```python
from build123d import *

# Parameters (mm, degrees)
SKETCH1_W                      = 42
SKETCH1_H                      = 42
BOSS_EXTRUDE1_DEPTH            = 22
CUT_EXTRUDE1_REACH             = 24
SKETCH2_R                      = 11.5
SKETCH2_R_2                    = 1.65
CUT_EXTRUDE1_DIRECTION_2_DEPTH = 1
CHAMFER1_SIZE                  = 4
SKETCH3_R                      = 3
CUT_EXTRUDE2_DEPTH             = 1
CUT_EXTRUDE2_DEPTH_BACK        = 5
CUT_EXTRUDE3_REACH             = 24
SKETCH4_R                      = 4.15
CUT_EXTRUDE3_DIRECTION_2_DEPTH = 1


with BuildPart() as part:
    # Sketch1 → Boss-Extrude1 (new body)
    with BuildSketch(Plane(origin=(0, 0, 0), x_dir=(1, 0, 0), z_dir=(0, 1, 0))):
        Rectangle(SKETCH1_W, SKETCH1_H)
    extrude(amount=BOSS_EXTRUDE1_DEPTH)

    # Sketch2 → Cut-Extrude1 (cut, up to next)
    with BuildSketch(Plane(origin=(0, 22, 0), x_dir=(1, 0, 0), z_dir=(0, 1, 0)), mode=Mode.PRIVATE) as cut_extrude1_sk1:
        Circle(SKETCH2_R)
    cut_extrude1_tool1 = extrude(cut_extrude1_sk1.sketch, amount=-CUT_EXTRUDE1_REACH, mode=Mode.PRIVATE) & part.part
    add(cut_extrude1_tool1.solids().sort_by_distance((0, 22, 0))[0], mode=Mode.SUBTRACT)
    # Sketch2 → Cut-Extrude1 (cut, up to next)
    with BuildSketch(Plane(origin=(0, 22, 0), x_dir=(1, 0, 0), z_dir=(0, 1, 0)), mode=Mode.PRIVATE) as cut_extrude1_sk2:
        with Locations((-15.5, 15)):
            Circle(SKETCH2_R_2)
    cut_extrude1_tool2 = extrude(cut_extrude1_sk2.sketch, amount=-CUT_EXTRUDE1_REACH, mode=Mode.PRIVATE) & part.part
    add(cut_extrude1_tool2.solids().sort_by_distance((-15.5, 22, -15))[0], mode=Mode.SUBTRACT)
    # Sketch2 → Cut-Extrude1 (cut, up to next)
    with BuildSketch(Plane(origin=(0, 22, 0), x_dir=(1, 0, 0), z_dir=(0, 1, 0)), mode=Mode.PRIVATE) as cut_extrude1_sk3:
        with Locations((15.5, 15)):
            Circle(SKETCH2_R_2)
    cut_extrude1_tool3 = extrude(cut_extrude1_sk3.sketch, amount=-CUT_EXTRUDE1_REACH, mode=Mode.PRIVATE) & part.part
    add(cut_extrude1_tool3.solids().sort_by_distance((15.5, 22, -15))[0], mode=Mode.SUBTRACT)
    # Sketch2 → Cut-Extrude1 (cut, up to next)
    with BuildSketch(Plane(origin=(0, 22, 0), x_dir=(1, 0, 0), z_dir=(0, 1, 0)), mode=Mode.PRIVATE) as cut_extrude1_sk4:
        with Locations((15.5, -15)):
            Circle(SKETCH2_R_2)
    cut_extrude1_tool4 = extrude(cut_extrude1_sk4.sketch, amount=-CUT_EXTRUDE1_REACH, mode=Mode.PRIVATE) & part.part
    add(cut_extrude1_tool4.solids().sort_by_distance((15.5, 22, 15))[0], mode=Mode.SUBTRACT)
    # Sketch2 → Cut-Extrude1 (cut, up to next)
    with BuildSketch(Plane(origin=(0, 22, 0), x_dir=(1, 0, 0), z_dir=(0, 1, 0)), mode=Mode.PRIVATE) as cut_extrude1_sk5:
        with Locations((-15.5, -15)):
            Circle(SKETCH2_R_2)
    cut_extrude1_tool5 = extrude(cut_extrude1_sk5.sketch, amount=-CUT_EXTRUDE1_REACH, mode=Mode.PRIVATE) & part.part
    add(cut_extrude1_tool5.solids().sort_by_distance((-15.5, 22, 15))[0], mode=Mode.SUBTRACT)

    # Sketch2 → Cut-Extrude1 direction 2 (cut)
    with BuildSketch(Plane(origin=(0, 22, 0), x_dir=(1, 0, 0), z_dir=(0, 1, 0))):
        Circle(SKETCH2_R)
        with Locations((-15.5, 15)):
            Circle(SKETCH2_R_2)
        with Locations((15.5, 15)):
            Circle(SKETCH2_R_2)
        with Locations((15.5, -15)):
            Circle(SKETCH2_R_2)
        with Locations((-15.5, -15)):
            Circle(SKETCH2_R_2)
    extrude(amount=CUT_EXTRUDE1_DIRECTION_2_DEPTH, mode=Mode.SUBTRACT)

    # Chamfer1
    chamfer1_edges = [part.edges().sort_by_distance(p)[0] for p in [
        (21, 11, 21),
        (-21, 11, 21),
        (-21, 11, -21),
        (21, 11, -21),
    ]]
    chamfer(chamfer1_edges, length=CHAMFER1_SIZE)

    # Sketch3 → Cut-Extrude2 (cut, two sides)
    with BuildSketch(Plane.XZ) as cut_extrude2_sk:
        with Locations((-15.5, 15)):
            Circle(SKETCH3_R)
        with Locations((15.5, 15)):
            Circle(SKETCH3_R)
        with Locations((15.5, -15)):
            Circle(SKETCH3_R)
        with Locations((-15.5, -15)):
            Circle(SKETCH3_R)
    extrude(amount=CUT_EXTRUDE2_DEPTH, mode=Mode.SUBTRACT)
    extrude(cut_extrude2_sk.sketch, amount=-CUT_EXTRUDE2_DEPTH_BACK, mode=Mode.SUBTRACT)

    # Sketch4 → Cut-Extrude3 (cut, up to next)
    with BuildSketch(Plane(origin=(0, 22, 0), x_dir=(1, 0, 0), z_dir=(0, 1, 0)), mode=Mode.PRIVATE) as cut_extrude3_sk1:
        with Locations((-21, 0)):
            Circle(SKETCH4_R)
    cut_extrude3_tool1 = extrude(cut_extrude3_sk1.sketch, amount=-CUT_EXTRUDE3_REACH, mode=Mode.PRIVATE) & part.part
    add(cut_extrude3_tool1.solids().sort_by_distance((-21, 22, 0))[0], mode=Mode.SUBTRACT)
    # Sketch4 → Cut-Extrude3 (cut, up to next)
    with BuildSketch(Plane(origin=(0, 22, 0), x_dir=(1, 0, 0), z_dir=(0, 1, 0)), mode=Mode.PRIVATE) as cut_extrude3_sk2:
        with Locations((21, 0)):
            Circle(SKETCH4_R)
    cut_extrude3_tool2 = extrude(cut_extrude3_sk2.sketch, amount=-CUT_EXTRUDE3_REACH, mode=Mode.PRIVATE) & part.part
    add(cut_extrude3_tool2.solids().sort_by_distance((21, 22, 0))[0], mode=Mode.SUBTRACT)

    # Sketch4 → Cut-Extrude3 direction 2 (cut)
    with BuildSketch(Plane(origin=(0, 22, 0), x_dir=(1, 0, 0), z_dir=(0, 1, 0))):
        with Locations((-21, 0)):
            Circle(SKETCH4_R)
        with Locations((21, 0)):
            Circle(SKETCH4_R)
    extrude(amount=CUT_EXTRUDE3_DIRECTION_2_DEPTH, mode=Mode.SUBTRACT)


solid = part.part
```
CAD build for the part. Positions are in the model's coordinates, mm. A direction names the side the tool comes from. Round coordinates to 2 decimals unless told otherwise and drop trailing zeros. Order: outer loops, then holes, each group sorted by start corner. A loop starts at its lowest first (then second) coordinate and runs counter-clockwise, first axis right, second up. Notation, with made-up numbers: (70, 56.5) -> (124, 56.5) arc R23 cw to (124, 81.5) -> close; hole circle Ø11 at (-5, 79). An arc over 180 degrees is marked (long way). One line per question, with ' | ' between items.
Q1. Two-plate mould, pull along Z, no slides. Class faces 3 (the cylindrical face through (17.074, 13.619, 14.504)), 4 (the flat face through (21, 11, -10)), 5 (the cylindrical face through (-13.926, 13.619, 14.504)), 6 (the flat face through (19, 11, -19)): released by +Z, released by -Z, zero draft, split by the parting line, or undercut.
Completed:
face 3: undercut | face 4: zero draft | face 5: undercut | face 6: released by -Z
Q2. Slice it at B-B (x = 0). Write the cut outline in (y, z), then the cut area to 3 significant figures.
Completed:
outline: (0, -21) -> (22, -21) -> (22, -11.5) -> (0, -11.5) -> close; (0, 11.5) -> (22, 11.5) -> (22, 21) -> (0, 21) -> close | area: 418 mm^2
Q3. Probe probe 1 along X at (y, z) = (14.25, 15); probe 2 along X at (y, z) = (5.5, -16.5); probe 3 along Z at (x, y) = (15, 12.25). List the from-to ranges inside material, lowest first.
Completed:
probe 1: x = -21 to -17.15, -13.85 to 13.85, 17.15 to 21 | probe 2: x = -21 to -16.19, -14.81 to 14.81, 16.19 to 21 | probe 3: z = -21 to -16.57, -13.43 to 13.43, 16.57 to 21
Q4. Slice it at A-A (z = 0). Write the cut outline in (x, y), then the cut area to 3 significant figures.
Completed:
outline: (-16.85, 0) -> (-11.5, 0) -> (-11.5, 22) -> (-16.85, 22) -> close; (11.5, 0) -> (16.85, 0) -> (16.85, 22) -> (11.5, 22) -> close | area: 235 mm^2
Q5. Slice it at D-D (x = 15.5). Write the cut outline in (y, z), then the cut area to 3 significant figures.
Completed:
outline: (0, -21) -> (22, -21) -> (22, -16.65) -> (5, -16.65) -> (5, -18) -> (0, -18) -> close; (0, -12) -> (5, -12) -> (5, -13.35) -> (22, -13.35) -> (22, 13.35) -> (5, 13.35) -> (5, 12) -> (0, 12) -> close; (0, 18) -> (5, 18) -> (5, 16.65) -> (22, 16.65) -> (22, 21) -> (0, 21) -> close | area: 752 mm^2
Q6. Drop flat-ended pins along their axis: pin 1 (3.5 mm diameter, centred on x = 15.5, z = -15, fed in from -Y); pin 2 (2 mm diameter, centred on x = -15.5, z = -15, fed in from +Y). Give the stop position or say it passes through.
Completed:
pin 1: stops at y = 5 | pin 2: passes through
Q7. Which spindle directions (+Z, -Z, +X, -X, +Y, -Y) get a long thin tool onto all of the face, cutting with end or side? Do faces 1 (the flat face through (-19, 11, 19)), 2 (the flat face through (17, 5, -16)). Say none if no direction does.
Completed:
face 1: +Z, -X, +Y, -Y | face 2: -Y
Q8. Slice it at C-C (y = 6.75). Write the cut outline in (x, z), then the cut area to 3 significant figures.
Completed:
outline: (-21, -17) -> (-17, -21) -> (17, -21) -> (21, -17) -> (21, -4.15) arc R4.15 cw to (21, 4.15) -> (21, 17) -> (17, 21) -> (-17, 21) -> (-21, 17) -> (-21, 4.15) arc R4.15 cw to (-21, -4.15) -> close; hole circle Ø3.3 at (-15.5, -15); hole circle Ø3.3 at (-15.5, 15); hole circle Ø23 at (0, 0); hole circle Ø3.3 at (15.5, -15); hole circle Ø3.3 at (15.5, 15) | area: 1,230 mm^2
